```python
from build123d import *

# Parameters (mm, degrees)
F0_W      = 156
F0_H      = 175
F1_DEPTH  = 1
F2_W      = 4.5
F2_H      = 175
F2_W_2    = 27
F2_H_2    = 149.5
F2_W_3    = 69
F2_H_3    = 82.25
F3_DEPTH  = 1.001
F4_W      = 15
F4_H      = 3
F5_DEPTH  = 1
F6_W      = 1
F6_H      = 19.1769432276
F6_H_2    = 19.2576229572
F7_DEPTH  = 2.75
F9_DEPTH  = 1
F10_W     = 1
F10_H     = 6
F11_DEPTH = 2.75
F12_W     = 1
F12_H     = 6
F13_DEPTH = 2.75


with BuildPart() as f1:
    # F0 (on Top) → F1 (new body)
    with BuildSketch(Plane.XY):
        with Locations((78, 87.5)):
            Rectangle(F0_W, F0_H)
    extrude(amount=F1_DEPTH)

    # F2 (on face) → F3 (cut, through all)
    with BuildSketch(Plane.XY.offset(1)):
        with Locations((2.25, 87.5)):
            Rectangle(F2_W, F2_H)
        with Locations((21, 80.75)):
            Rectangle(F2_W_2, F2_H_2)
        with Locations((78, 130.875)):
            Rectangle(F2_W_3, F2_H_3)
        with Locations((78, 44.125)):
            Rectangle(F2_W_3, F2_H_3)
        with Locations((135, 94.25)):
            Rectangle(F2_W_2, F2_H_2)
        with Locations((153.75, 87.5)):
            Rectangle(F2_W, F2_H)
    extrude(amount=-F3_DEPTH, mode=Mode.SUBTRACT)

    # F4 (on face) → F5 (join)
    with BuildSketch(Plane.XY.offset(1)):
        Polygon((24.5, 155.5), (24.5, 175), (5.5, 175), (5.5, 155.5), (7.5, 155.5), align=None)
        with Locations((61.5, 173.5)):
            Rectangle(F4_W, F4_H)
        with Locations((94.5, 173.5)):
            Rectangle(F4_W, F4_H)
        Polygon((131.5, 0), (150.5, 0), (150.5, 19.5), (148.5, 19.5), (131.5, 19.5), align=None)
        with Locations((94.5, 1.5)):
            Rectangle(F4_W, F4_H)
        with Locations((61.5, 1.5)):
            Rectangle(F4_W, F4_H)
    extrude(amount=F5_DEPTH)

    # F6 (on face) → F7 (join)
    with BuildSketch(Plane.XY.offset(1)):
        with Locations((151, 9.5884716138)):
            Rectangle(F6_W, F6_H)
        with Locations((5, 165.3711885214)):
            Rectangle(F6_W, F6_H_2)
    extrude(amount=F7_DEPTH)

    # F8 (on face) → F9 (join)
    with BuildSketch(Plane.XY.offset(1)):
        Polygon((5.5, 0), (24.5, 0), (24.5, 6), (7.5, 6), (5.5, 6), align=None)
        Polygon((131.5, 175), (131.5, 169), (148.5, 169), (150.5, 169), (150.5, 175), align=None)
    extrude(amount=F9_DEPTH)

    # F10 (on face) → F11 (join)
    with BuildSketch(Plane.XY.offset(1)):
        with Locations((151, 172)):
            Rectangle(F10_W, F10_H)
    extrude(amount=F11_DEPTH)

    # F12 (on face) → F13 (join)
    with BuildSketch(Plane.XY.offset(1)):
        with Locations((5, 3)):
            Rectangle(F12_W, F12_H)
    extrude(amount=F13_DEPTH)


solid = f1.part
```
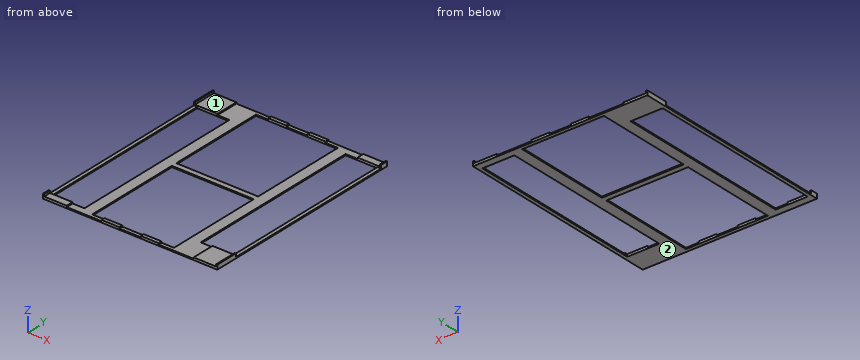
CAD build for the part. Positions are in the model's coordinates, mm. Face numbers are marked on the shaded views. Coordinates: 2 decimals unless noted, no trailing zeros. Order: outer loops, then holes, each group sorted by start corner. A loop starts at its lowest first (then second) coordinate and runs counter-clockwise, first axis right, second up. Notation, with made-up numbers: (41, -2) -> (49, -2) arc R15 ccw to (49, 14) -> close; hole circle Ø4 at (56.5, -0.5). An arc over 180 degrees is marked (long way). Use one line per item in the form item = value. Start each with the question number.
1) Band-saw the part on C-C on z = 2.7. Give the cut face in (x, y), then the cut area to 3 significant figures.
2) Band-saw the part on B-B on x = 127. Give the cut face in (y, z), then the cut area to 3 significant figures.
3) Drill centre lines: L1, parallel to X at y = 47, z = 0.4; L2, parallel to X at y = 166.5, z = 0.9; L3, parallel to Y at x = 92, z = 0.4. Where is each one in solid material? Low to high. Write a range as [from, to].
4) Pull direction X, two halves, no side cores. Call the marked faces 1 and 2: +X half, -X half, draft (parallel to the pull), parting line (faces both ways), or undercut.
5) Drop flat-ended pins along their axis: pin 1 (3.5 mm diameter, centred on x = 75.5, y = 173, fed in from +Z); pin 2 (2 mm diameter, centred on y = 27, z = 3, fed in from -X); pin 3 (0.9 mm diameter, centred on y = 164, z = 3, fed in from +X); pin 4 (1.4 mm diameter, centred on y = 7, z = 3, fed in from -X). Give the stop position or say it passes through.
6) Band-saw the part on D-D on x = 45.5. Give the cut face in (y, z), then the cut area to 3 significant figures.
7) Band-saw the part on A-A on y = 94. Give the cut face in (x, z), then the cut area to 3 significant figures.
Entries:
q1.outline = (4.5, 0) -> (5.5, 0) -> (5.5, 6) -> (4.5, 6) -> close; (4.5, 155.74) -> (5.5, 155.74) -> (5.5, 175) -> (4.5, 175) -> close; (150.5, 0) -> (151.5, 0) -> (151.5, 19.18) -> (150.5, 19.18) -> close; (150.5, 169) -> (151.5, 169) -> (151.5, 175) -> (150.5, 175) -> close
q1.area = 50.4 mm2
q2.outline = (0, 0) -> (19.5, 0) -> (19.5, 1) -> (0, 1) -> close; (169, 0) -> (175, 0) -> (175, 1) -> (169, 1) -> close
q2.area = 25.5 mm2
q3.L1 = [4.5, 7.5], [34.5, 43.5], [112.5, 121.5], [148.5, 151.5]
q3.L2 = [4.5, 43.5], [112.5, 121.5], [148.5, 151.5]
q3.L3 = [0, 3], [85.25, 89.75], [172, 175]
q4.face_1 = undercut
q4.face_2 = draft
q5.pin_1 = 1
q5.pin_2 = through
q5.pin_3 = 5.5
q5.pin_4 = 150.5
q6.outline = (0, 0) -> (3, 0) -> (3, 1) -> (0, 1) -> close; (85.25, 0) -> (89.75, 0) -> (89.75, 1) -> (85.25, 1) -> close; (172, 0) -> (175, 0) -> (175, 1) -> (172, 1) -> close
q6.area = 10.5 mm2
q7.outline = (4.5, 0) -> (7.5, 0) -> (7.5, 1) -> (4.5, 1) -> close; (34.5, 0) -> (43.5, 0) -> (43.5, 1) -> (34.5, 1) -> close; (112.5, 0) -> (121.5, 0) -> (121.5, 1) -> (112.5, 1) -> close; (148.5, 0) -> (151.5, 0) -> (151.5, 1) -> (148.5, 1) -> close
q7.area = 24.0 mm2
